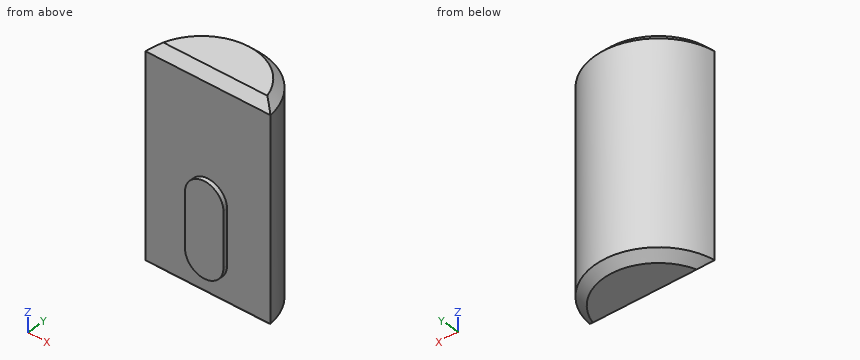
from build123d import *

# Parameters (mm, degrees)
PAD010_DEPTH    = 10
CHAMFER005_SIZE = 0.4
PAD011_DEPTH    = 0.2


with BuildPart() as body009:
    # Sketch023 → Pad010 (new body)
    with BuildSketch(Plane.XY):
        with BuildLine():
            ThreePointArc((-2.929164, -0.35), (0, -2.95), (2.929164, -0.35))
            Line((-2.929164, -0.35), (2.929164, -0.35))
        make_face()
    extrude(amount=-PAD010_DEPTH)

    # Chamfer005
    chamfer005_edges = [body009.edges().sort_by_distance(p)[0] for p in [
        (0, -2.95, 0),
        (0, -0.35, 0),
        (0, -2.95, -10),
        (0, -0.35, -10),
    ]]
    chamfer(chamfer005_edges, length=CHAMFER005_SIZE)

    # Sketch024 (on Face2 of Chamfer005) → Pad011 (join)
    with BuildSketch(Plane(origin=(0, -0.35, 0), x_dir=(-1, 0, 0), z_dir=(0, 1, 0))):
        with BuildLine():
            ThreePointArc((0.9, -5.5), (0, -4.6), (-0.9, -5.5))
            Line((-0.9, -5.5), (-0.9, -8))
            ThreePointArc((-0.9, -8), (0, -8.9), (0.9, -8))
            Line((0.9, -5.5), (0.9, -8))
        make_face()
    extrude(amount=PAD011_DEPTH)


with BuildPart() as holder2:
    # Part__Mirroring: instance of Body009
    add(body009.part.mirror(Plane(origin=(0, 0, 0), x_dir=(1, 0, 0), z_dir=(0, 1, 0))))


solid = holder2.part
Work out the finished part from the listing and answer in its coordinate system (mm). Round coordinates to 2 decimals unless told otherwise and drop trailing zeros. Write each loop counter-clockwise with the first axis right and the second up, starting at its lowest first coordinate (ties: lowest second). Pieces come first, ordered by that corner, then holes. Notation, with made-up numbers: M -7,-38 L 46,-38 A24 ccw 46,-24 Z; hole C 17,75.25 d11. An arc over 180 degrees is marked long. Use a Markdown table: item, result.
1) The part is cut by section D-D on z = -5.25. Give the vertices of the cut face in (x, y).
Taken from the geometry:
| item | result |
|---|---|
| outline | M -2.93,0.35 L -0.86,0.35 L -0.86,0.15 L 0.86,0.15 L 0.86,0.35 L 2.93,0.35 A2.95 ccw Z |
2) The part is cut by section C-C on z = -8.5. Give the vertices of the cut face in (x, y), plus the area to 3 significant figures.
Taken from the geometry:
| item | result |
|---|---|
| outline | M -2.93,0.35 L -0.75,0.35 L -0.75,0.15 L 0.75,0.15 L 0.75,0.35 L 2.93,0.35 A2.95 ccw Z |
| area | 11.9 mm2 |
3) The part is cut by section A-A on x = 0. Give the vertices of the cut face in (y, z).
Taken from the geometry:
| item | result |
|---|---|
| outline | M 0.15,-8.9 L 0.35,-8.9 L 0.35,-9.6 L 0.75,-10 L 2.55,-10 L 2.95,-9.6 L 2.95,-0.4 L 2.55,0 L 0.75,0 L 0.35,-0.4 L 0.35,-4.6 L 0.15,-4.6 Z |
4) The part is cut by section B-B on z = -2.5. Give the vertices of the cut face in (x, y), plus the area to 3 significant figures.
Taken from the geometry:
| item | result |
|---|---|
| outline | M -2.93,0.35 L 2.93,0.35 A2.95 ccw Z |
| area | 11.6 mm2 |
5) Consider line 1 (Y direction, x = -0.05, z = -0.5); line 2 (Z direction, x = 1.7, y = 0.7); line 3 (X direction, y = 2.55, z = -6). Determine where each line is inside the solid, lowest interval first. Write a range as [from, to].
Taken from the geometry:
| item | result |
|---|---|
| line 1 | y = [0.35, 2.95] |
| line 2 | z = [-9.95, -0.05] |
| line 3 | x = [-1.48, 1.48] |
